Geometry: final body of the model. Coordinates: model frame, mm. Face numbers are marked on the shaded views. A direction names the side the tool comes from. Coordinates: 2 decimals unless noted, no trailing zeros. Order: outer loops, then holes, each group sorted by start corner. A loop starts at its lowest first (then second) coordinate and runs counter-clockwise, first axis right, second up. Notation, with made-up numbers: M 20.5,77 L 26.5,77 A23 cw 26.5,98 Z; hole C -25.75,30 d8. An arc over 180 degrees is marked long. Write item = value, one per line. Start each with the question number.
```python
from build123d import *

# Parameters (mm, degrees)
BOX001_W        = 200
BOX001_H        = 30
BOX001_DEPTH    = 30
SKETCH003_W     = 207.751177
SKETCH003_H     = 24
POCKET005_DEPTH = 27
POCKET001_DEPTH = 50
SKETCH006_R     = 3
POCKET003_DEPTH = 50
SKETCH004_R     = 3
POCKET004_DEPTH = 5


with BuildPart() as part:
    # Box001 → Box001 (join)
    with BuildSketch(Plane.XY):
        with Locations((100, 15)):
            Rectangle(BOX001_W, BOX001_H)
    extrude(amount=BOX001_DEPTH)

    # Sketch003 (on Face6 of Box001) → Pocket005 (cut)
    with BuildSketch(Plane.XY.offset(30)):
        with Locations((99.970328, 15)):
            Rectangle(SKETCH003_W, SKETCH003_H)
    extrude(amount=-POCKET005_DEPTH, mode=Mode.SUBTRACT)

    # Sketch005 (on Face9 of Pocket005) → Pocket001 (cut)
    with BuildSketch(Plane.XZ):
        Polygon((20.202248, 34.020094), (202.686674, 3.393335), (216.979173, 34.020094), align=None)
    extrude(amount=-POCKET001_DEPTH, mode=Mode.SUBTRACT)

    # Sketch006 → Pocket003 (cut)
    with BuildSketch(Plane.XZ):
        with Locations((15, 15)):
            Circle(SKETCH006_R)
    extrude(amount=-POCKET003_DEPTH, mode=Mode.SUBTRACT)

    # Sketch004 (on Face4 of Pocket001) → Pocket004 (cut)
    with BuildSketch(Plane.XY.offset(3)):
        with Locations((45, 15)):
            Circle(SKETCH004_R)
        with Locations((170, 15)):
            Circle(SKETCH004_R)
    extrude(amount=-POCKET004_DEPTH, mode=Mode.SUBTRACT)


with BuildPart() as part_1:
    # Body003 placement: moved
    add(part.part.moved(Location((150, 135, 30))))


solid = part_1.part
```
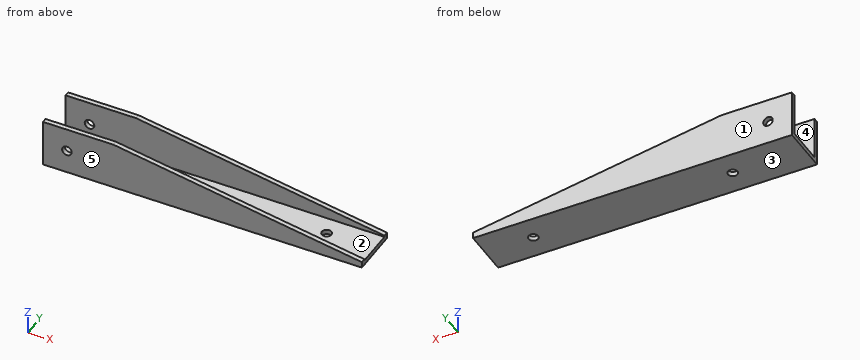
Item 1: Section query C-C on z = 45. Output: boundary loops of the cut face in (x, y), and give its area (3 significant figures).
Item 2: Section query B-B on x = 320. Output: boundary loops of the cut face in (y, z).
Item 3: Reachability of the marked faces 4 and 5 from +Z, -Z, +X, -X, +Y, -Y: full face, straight path, thin tool, end or side. Return the list, or none.
Item 4: Section query A-A on x = 165. Output: boundary loops of the cut face in (y, z).
Item 5: Material intervals for probe 1 along Z at (x, y) = (165, 136.1); probe 2 along Y at (x, z) = (193, 57.75); probe 3 along X at (y, z) = (150, 30.7), sorted ascending. Write a range as [from, to].
Item 6: Draft query along Y for the marked faces 1, 2 and 3. Return one class per face: pulls with the +Y half, pulls with the -Y half, needs draft (parallel to the pull), parting line crosses it, or undercut.
Item 7: First-contact query: pin 1 (10 mm diameter, centred on x = 239.5, y = 160.5, fed in from +Z); pin 2 (6 mm diameter, centred on y = 157, z = 36.5, fed in from +X); pin 3 (1.5 mm diameter, centred on x = 301, y = 138, fed in from +Z); pin 4 (9.5 mm diameter, centred on x = 320, y = 150, fed in from +Z). Flat tips, straight axial feed; report the tip coordinate or a pass-through.
Item 8: Section query D-D on z = 36.5. Output: boundary loops of the cut face in (x, y).
Ans:
q1.outline = M 150,135 L 162,135 L 162,138 L 150,138 Z; M 150,162 L 162,162 L 162,165 L 150,165 Z; M 168,135 L 283.53,135 L 283.53,138 L 168,138 Z; M 168,162 L 283.53,162 L 283.53,165 L 168,165 Z
q1.area = 765 mm^2
q2.outline = M 135,30 L 147,30 L 147,33 L 138,33 L 138,38.88 L 135,38.88 Z; M 153,30 L 165,30 L 165,38.88 L 162,38.88 L 162,33 L 153,33 Z
q3.face_4 = +Z, +X, -X
q3.face_5 = +Z, -Z, +X, -X, -Y
q4.outline = M 135,30 L 165,30 L 165,42 L 162,42 L 162,33 L 138,33 L 138,42 L 135,42 Z; M 135,48 L 138,48 L 138,60 L 135,60 Z; M 162,48 L 165,48 L 165,60 L 162,60 Z
q5.probe_1 = [30, 42], [48, 60]
q5.probe_2 = [135, 138], [162, 165]
q5.probe_3 = [150, 192], [198, 317], [323, 350]
q6.face_1 = pulls with the +Y half
q6.face_2 = undercut
q6.face_3 = needs draft
q7.pin_1 = 53.19
q7.pin_2 = through
q7.pin_3 = 42.19
q7.pin_4 = 33
q8.outline = M 150,135 L 334.18,135 L 334.18,138 L 150,138 Z; M 150,162 L 334.18,162 L 334.18,165 L 150,165 Z
